Drawing for the job (mm, zero at the part's lowest x, y, z). Coordinates: 2 decimals unless noted, no trailing zeros. Order: outer loops, then holes, each group sorted by start corner. A loop starts at its lowest first (then second) coordinate and runs counter-clockwise, first axis right, second up.
1) Pin check, flat tips, straight feed: pin 1 Ø4.5 at (x, y) = (10, 10) entering from +Z; pin 2 Ø12 at (x, y) = (130.5, 65) entering from -Z; pin 3 Ø8.5 at (x, y) = (250, 10) entering from +Z. Stop position of each tip, or through.
2) Cut at B-B (x = 10). List the corners of the cut face in (y, z) (3 decimals).
3) Wall check: L1, parallel to Y at x = 10, z = 1.9 (3 decimals); L2, parallel to X at y = 10, z = 1.6 (3 decimals); L3, parallel to Y at x = 249.5, z = 7.75. Give the ranges that are in metal, low to high.
4) Cut at A-A (y = 10). List the corners of the cut face in (x, z) (3 decimals).
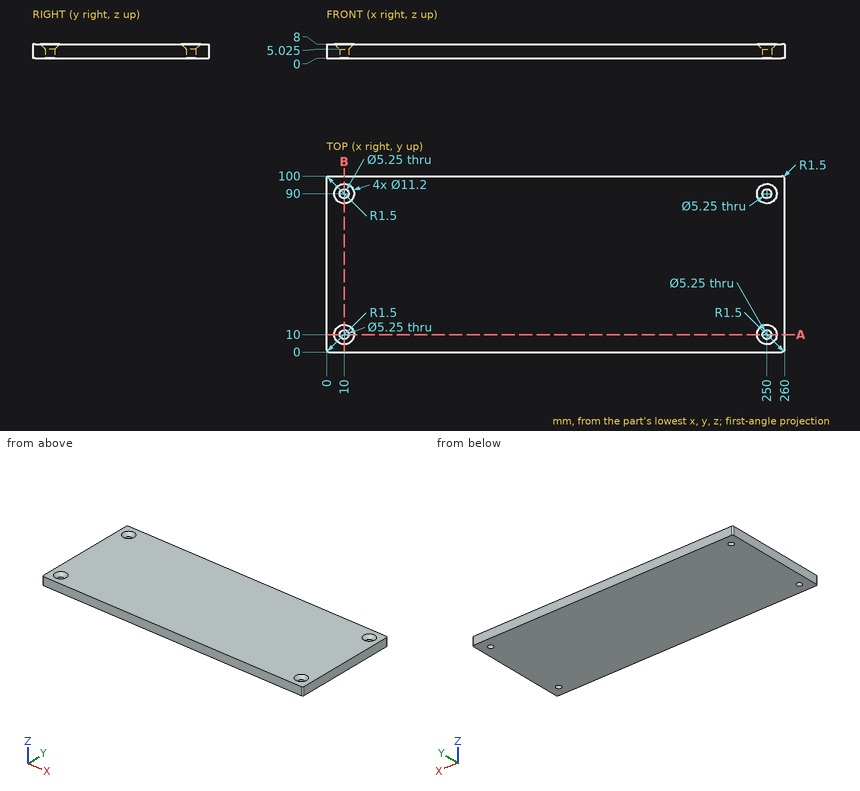
Geometry check:
1. pin 1: passes through
1. pin 2: stops at z = 0
1. pin 3: stops at z = 6.65
2. outline: (0, 0) - (7.375, 0) - (7.375, 5.025) - (4.4, 8) - (0, 8) - close; (12.625, 0) - (87.375, 0) - (87.375, 5.025) - (84.4, 8) - (15.6, 8) - (12.625, 5.025) - close; (92.625, 0) - (100, 0) - (100, 8) - (95.6, 8) - (92.625, 5.025) - close
3. L1: y = 0 to 7.375, 12.625 to 87.375, 92.625 to 100
3. L2: x = 0 to 7.375, 12.625 to 247.375, 252.625 to 260
3. L3: y = 0 to 4.67, 15.33 to 84.67, 95.33 to 100
4. outline: (0, 0) - (7.375, 0) - (7.375, 5.025) - (4.4, 8) - (0, 8) - close; (12.625, 0) - (247.375, 0) - (247.375, 5.025) - (244.4, 8) - (15.6, 8) - (12.625, 5.025) - close; (252.625, 0) - (260, 0) - (260, 8) - (255.6, 8) - (252.625, 5.025) - close
